Geometry check sheet. Reference: the model listing, model coordinates, mm. Face numbers are marked on the shaded views. A direction names the side the tool comes from. Coordinates: 2 decimals unless noted, no trailing zeros. Order: outer loops, then holes, each group sorted by start corner. A loop starts at its lowest first (then second) coordinate and runs counter-clockwise, first axis right, second up. Notation, with made-up numbers: (70.25, 60.5) -> (126.25, 60.5) arc R12 ccw to (126.25, 79.5) -> close; hole circle Ø2 at (34, 20.25). An arc over 180 degrees is marked (long way). Answer as CSV lines item,"result". Start each with the question number.
from build123d import *

# Parameters (mm, degrees)
SKETCH1_W           = 14
SKETCH1_H           = 14
BOSS_EXTRUDE1_DEPTH = 4
SKETCH2_W           = 25
SKETCH2_H           = 25
SKETCH2_R           = 1.2446
BOSS_EXTRUDE2_DEPTH = 10
SKETCH3_R           = 4.23
CUT_EXTRUDE1_DEPTH  = 9.8
SKETCH5_R           = 0.6604
CUT_EXTRUDE2_DEPTH  = 14
SKETCH8_R           = 0.85
CUT_EXTRUDE3_DEPTH  = 4


with BuildPart() as part:
    # Sketch1 → Boss-Extrude1 (new body)
    with BuildSketch(Plane(origin=(0, 0, 0), x_dir=(1, 0, 0), z_dir=(0, 1, 0))):
        Rectangle(SKETCH1_W, SKETCH1_H)
    extrude(amount=BOSS_EXTRUDE1_DEPTH)

    # Sketch2 → Boss-Extrude2 (add)
    with BuildSketch(Plane.XZ):
        Rectangle(SKETCH2_W, SKETCH2_H)
        with Locations((-9.75, 9.75)):
            Circle(SKETCH2_R, mode=Mode.SUBTRACT)
        with Locations((9.75, 9.75)):
            Circle(SKETCH2_R, mode=Mode.SUBTRACT)
        with Locations((9.75, -9.75)):
            Circle(SKETCH2_R, mode=Mode.SUBTRACT)
        with Locations((-9.75, -9.75)):
            Circle(SKETCH2_R, mode=Mode.SUBTRACT)
    extrude(amount=BOSS_EXTRUDE2_DEPTH)

    # Sketch3 → Cut-Extrude1 (cut)
    with BuildSketch(Plane.XZ.offset(10)):
        Circle(SKETCH3_R)
    extrude(amount=-CUT_EXTRUDE1_DEPTH, mode=Mode.SUBTRACT)

    # Sketch4 → Revolve1 (revolve)
    with BuildSketch(Plane(origin=(0, 0, 0), x_dir=(0, 0, -1), z_dir=(1, 0, 0))):
        Polygon((0.6604, 11), (0.6604, 4), (1.6, 4), (1.6, 10.5), (1.1, 11), align=None)
    revolve(axis=Axis((0, 4, 0), (0, 1, 0)))

    # Sketch5 → Cut-Extrude2 (cut)
    with BuildSketch(Plane(origin=(0, 4, 0), x_dir=(1, 0, 0), z_dir=(0, 1, 0))):
        Circle(SKETCH5_R)
    extrude(amount=-CUT_EXTRUDE2_DEPTH, mode=Mode.SUBTRACT)

    # Sketch8 → Cut-Extrude3 (cut)
    with BuildSketch(Plane(origin=(0, 11, 0), x_dir=(1, 0, 0), z_dir=(0, 1, 0))):
        with Locations((1.334621812, 0)):
            Circle(SKETCH8_R)
    extrude(amount=-CUT_EXTRUDE3_DEPTH, mode=Mode.SUBTRACT)


solid = part.part
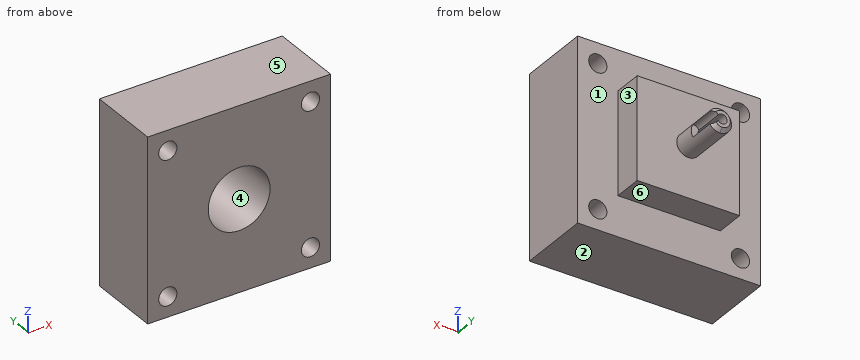
Q1. Sectioned sample at B-B, the plane x = -9.75. Record the cut outline in (y, z).
Q2. Release check for a two-part mould opening along Z. For the marked faces 3, 4, 5 and 6 record: released by +Z, released by -Z, zero draft, split by the parting line, or undercut.
Q3. Go/stop test with flat-tipped pins: pin 1 Ø3 at (y, z) = (2.5, 2.5) entering from -X; pin 2 Ø7.5 at (x, z) = (0, 0) entering from -Y; pin 3 Ø3 at (x, z) = (-9.75, 9.75) entering from +Y; pin 4 Ø7.5 at (x, z) = (4.5, 0) entering from +Y. Record where each tip stops, or that it passes through.
Q4. Sectioned sample at C-C, the plane z = 9.75. Record the cut outline in (x, y), then the cut area to 3 significant figures.
Q5. Sectioned sample at D-D, the plane z = 0. Record the cut outline in (x, y).
Q6. Sectioned sample at A-A, the plane y = -5.25. Record the cut outline in (x, z), then the cut area to 3 significant figures.
Q7. Access from +Z, -Z, +X, -X, +Y, -Y to the whole of each face (thin tool, end or side, straight path). Record for the marked faces 1 and 2.
Q8. Thickness scan on L1, parallel to Z at x = -9.75, y = -6; L2, parallel to X at y = 2.45, z = 0. Record the ranges inside material, lowest first.
Geometry results:
1,outline,"(-10, -12.5) -> (0, -12.5) -> (0, -10.99) -> (-10, -10.99) -> close; (-10, -8.51) -> (0, -8.51) -> (0, 8.51) -> (-10, 8.51) -> close; (-10, 10.99) -> (0, 10.99) -> (0, 12.5) -> (-10, 12.5) -> close"
2,face 3,"zero draft"
2,face 4,"undercut"
2,face 5,"released by +Z"
2,face 6,"released by -Z"
3,pin 1,"stops at x = -7"
3,pin 2,"stops at y = -0.2"
3,pin 3,"stops at y = 0"
3,pin 4,"stops at y = 11"
4,outline,"(-12.5, -10) -> (-10.99, -10) -> (-10.99, 0) -> (-12.5, 0) -> close; (-8.51, -10) -> (8.51, -10) -> (8.51, 0) -> (-8.51, 0) -> close; (10.99, -10) -> (12.5, -10) -> (12.5, 0) -> (10.99, 0) -> close"
4,area,"200 mm^2"
5,outline,"(-12.5, -10) -> (-4.23, -10) -> (-4.23, -0.2) -> (-0.66, -0.2) -> (-0.66, 11) -> (-1.1, 11) -> (-1.6, 10.5) -> (-1.6, 4) -> (-7, 4) -> (-7, 0) -> (-12.5, 0) -> close; (0.66, -0.2) -> (4.23, -0.2) -> (4.23, -10) -> (12.5, -10) -> (12.5, 0) -> (7, 0) -> (7, 4) -> (1.6, 4) -> (1.6, 7) -> (0.66, 7) -> close"
6,outline,"(-12.5, -12.5) -> (12.5, -12.5) -> (12.5, 12.5) -> (-12.5, 12.5) -> close; hole circle Ø2.49 at (-9.75, -9.75); hole circle Ø2.49 at (-9.75, 9.75); hole circle Ø8.46 at (0, 0); hole circle Ø2.49 at (9.75, -9.75); hole circle Ø2.49 at (9.75, 9.75)"
6,area,"549 mm^2"
7,face 1,"+Y"
7,face 2,"-Z, +X, -X, +Y, -Y"
8,L1,"z = -12.5 to -10.99, -8.51 to 8.51, 10.99 to 12.5"
8,L2,"x = -7 to -0.66, 0.66 to 7"
